from build123d import *

# Parameters (mm, degrees)
F0_R     = 15.875
F0_R_2   = 4.826
F1_DEPTH = 25.4


with BuildPart() as f1:
    # F0 (on Front) → F1 (new body)
    with BuildSketch(Plane.XZ):
        Circle(F0_R)
        with BuildLine():
            ThreePointArc((4.891009, 11.720411), (10.56896, 7.04181), (12.7, 0))
            ThreePointArc((12.7, 0), (12.291071, -3.196806), (11.09062, -6.187743))
            ThreePointArc((11.09062, -6.187743), (6.430617, -10.951583), (0, -12.7))
            ThreePointArc((0, -12.7), (-3.046434, -12.329203), (-5.914977, -11.238463))
            ThreePointArc((-5.914977, -11.238463), (-10.872217, -6.563908), (-12.7, 0))
            ThreePointArc((-12.7, 0), (-12.429648, 2.606501), (-11.630103, 5.10203))
            ThreePointArc((-11.630103, 5.10203), (-6.946014, 10.632163), (0, 12.7))
            ThreePointArc((0, 12.7), (2.494071, 12.452695), (4.891009, 11.720411))
        make_face(mode=Mode.SUBTRACT)
        with BuildLine():
            Line((2.281079, 5.926144), (4.891009, 11.720411))
            ThreePointArc((4.891009, 11.720411), (2.494071, 12.452695), (0, 12.7))
            Line((0, 12.7), (0, 6.35))
            ThreePointArc((0, 6.35), (1.160062, 6.243137), (2.281079, 5.926144))
        make_face()
        with BuildLine():
            Line((-5.833724, 2.508019), (-11.630103, 5.10203))
            ThreePointArc((-11.630103, 5.10203), (-12.429648, 2.606501), (-12.7, 0))
            Line((-12.7, 0), (-6.35, 0))
            ThreePointArc((-6.35, 0), (-6.219592, 1.280303), (-5.833724, 2.508019))
        make_face()
        with BuildLine():
            ThreePointArc((-5.914977, -11.238463), (-3.046434, -12.329203), (0, -12.7))
            Line((0, -12.7), (0, -6.35))
            ThreePointArc((0, -6.35), (-1.77968, -6.09551), (-3.416711, -5.352437))
            Line((-3.416711, -5.352437), (-5.914977, -11.238463))
        make_face()
        with BuildLine():
            ThreePointArc((11.09062, -6.187743), (12.291071, -3.196806), (12.7, 0))
            Line((12.7, 0), (6.35, 0))
            ThreePointArc((6.35, 0), (6.129141, -1.660162), (5.481926, -3.204839))
            Line((5.481926, -3.204839), (11.09062, -6.187743))
        make_face()
        with BuildLine():
            ThreePointArc((5.481926, -3.204839), (6.129141, -1.660162), (6.35, 0))
            ThreePointArc((6.35, 0), (5.234852, 3.594276), (2.281079, 5.926144))
            ThreePointArc((2.281079, 5.926144), (1.160062, 6.243137), (0, 6.35))
            ThreePointArc((0, 6.35), (-3.492605, 5.303226), (-5.833724, 2.508019))
            ThreePointArc((-5.833724, 2.508019), (-6.219592, 1.280303), (-6.35, 0))
            ThreePointArc((-6.35, 0), (-5.5686, -3.051752), (-3.416711, -5.352437))
            ThreePointArc((-3.416711, -5.352437), (-1.77968, -6.09551), (0, -6.35))
            ThreePointArc((0, -6.35), (3.160045, -5.507868), (5.481926, -3.204839))
        make_face()
        Circle(F0_R_2, mode=Mode.SUBTRACT)
    extrude(amount=F1_DEPTH)


solid = f1.part
Read the model definition and answer for the solid it produces. Units are mm, in the model's axes. Coordinates: 2 decimals unless noted, no trailing zeros. Order: outer loops, then holes, each group sorted by start corner. A loop starts at its lowest first (then second) coordinate and runs counter-clockwise, first axis right, second up. Notation, with made-up numbers: (14, 61) - (60, 61) arc R23 cw to (60, 76) - close; hole circle Ø1 at (81, -38). An arc over 180 degrees is marked (long way). Use one line per item in the form item = value.
(1) Section A-A, the plane z = 3.5 is taken. Give the vertices of the cut face in (x, y).
Computed values:
outline = (-15.48, -25.4) - (-8.05, -25.4) - (-8.05, 0) - (-15.48, 0) - close; (-5.3, -25.4) - (-3.32, -25.4) - (-3.32, 0) - (-5.3, 0) - close; (3.32, -25.4) - (5.3, -25.4) - (5.3, 0) - (3.32, 0) - close; (12.21, -25.4) - (15.48, -25.4) - (15.48, 0) - (12.21, 0) - close
(2) Given pin 1 Ø1 at (x, y) = (12.5, -11) entering from +Z; pin 2 Ø1.9 at (y, z) = (-19, -10) entering from +X; pin 3 Ø12 at (y, z) = (-4.5, -7) entering from +X; pin 4 Ø1.5 at (x, z) = (8, -7.5) entering from -Y, each flat-ended and moving along its own axis, determine where each tip first touches the part or whether it passes through.
Computed values:
pin_1 = 10.39
pin_2 = 13.04
pin_3 = 15.84
pin_4 = through
(3) Section D-D, the plane x = 7 is taken. Give the vertices of the cut face in (y, z).
Computed values:
outline = (-25.4, -14.25) - (0, -14.25) - (0, -10.6) - (-25.4, -10.6) - close; (-25.4, -4.01) - (0, -4.01) - (0, 0) - (-25.4, 0) - close; (-25.4, 10.6) - (0, 10.6) - (0, 14.25) - (-25.4, 14.25) - close
(4) Section C-C, the plane z = 7.5 is taken. Give the vertices of the cut face in (x, y), then the cut area to 3 significant figures.
Computed values:
outline = (-13.99, -25.4) - (-10.25, -25.4) - (-10.25, 0) - (-13.99, 0) - close; (0, -25.4) - (2.99, -25.4) - (2.99, 0) - (0, 0) - close; (10.25, -25.4) - (13.99, -25.4) - (13.99, 0) - (10.25, 0) - close
area = 266 mm²
(5) Straight lines are drawn through the part: L1, parallel to Z at x = 2.5, y = -10.5; L2, parallel to Z at x = -8, y = -15.75; L3, parallel to Z at x = -10, y = -7.25. For each, find the intervals that lie inside material, in ascending order.
Computed values:
L1 = -15.68 to -12.45, -5.84 to -4.13, 4.13 to 5.84, 6.41 to 15.68
L2 = -13.71 to -9.86, 0 to 3.48, 9.86 to 13.71
L3 = -12.33 to -7.83, 0 to 4.37, 7.83 to 12.33
(6) For a pull along Z with two mould halves and no side action, classify faces 1 (the face through (-3.441, -12.522, -15.497)), 2 (the face through (10.51, -12.52, 7.13)), 3 (the face through (-4, 0, -3)) as pulls with the +Z half, pulls with the -Z half, needs draft (parallel to the pull), parting line crosses it, or undercut.
Computed values:
face_1 = parting line crosses it
face_2 = undercut
face_3 = needs draft
(7) Section B-B, the plane y = -22.25 is taken. Give the vertices of the cut face in (x, z) (3 decimals), then the cut area to 3 significant figures.
Computed values:
outline = circle Ø31.75 at (0, 0); hole (-12.7, 0) arc R12.7 ccw to (-5.915, -11.238) - (-3.417, -5.352) arc R6.35 cw to (-6.35, 0) - close; hole (-11.63, 5.102) - (-5.834, 2.508) arc R6.35 cw to (0, 6.35) - (0, 12.7) arc R12.7 ccw to start; hole circle Ø9.652 at (0, 0); hole (0, -12.7) arc R12.7 ccw to (11.091, -6.188) - (5.482, -3.205) arc R6.35 cw to (0, -6.35) - close; hole (2.281, 5.926) arc R6.35 cw to (6.35, 0) - (12.7, 0) arc R12.7 ccw to (4.891, 11.72) - close
area = 449 mm²
